```python
from build123d import *

# Parameters (mm, degrees)
SKETCH1_W           = 61
SKETCH1_H           = 10
SKETCH1_R           = 1.5
BOSS_EXTRUDE1_DEPTH = 5
SKETCH2_W           = 3
SKETCH2_H           = 10
BOSS_EXTRUDE2_DEPTH = 45
SKETCH3_R           = 1.75
CUT_EXTRUDE1_DEPTH  = 80.072172407
SKETCH4_W           = 15
SKETCH4_H           = 6
BOSS_EXTRUDE3_DEPTH = 3
SKETCH5_R           = 1.75
CUT_EXTRUDE2_DEPTH  = 82.52017035
SKETCH6_W           = 61
SKETCH6_H           = 10
SKETCH6_R           = 1.5
BOSS_EXTRUDE4_DEPTH = 5
SKETCH7_R           = 1.75
CUT_EXTRUDE3_DEPTH  = 85.679030308
SKETCH8_W           = 61
SKETCH8_H           = 55
SKETCH8_W_2         = 55
SKETCH8_H_2         = 45
BOSS_EXTRUDE5_DEPTH = 10
SKETCH13_R          = 1.7
CUT_EXTRUDE5_DEPTH  = 18


with BuildPart() as part:
    # Sketch1 → Boss-Extrude1 (new body)
    with BuildSketch(Plane(origin=(0, 0, 0), x_dir=(1, 0, 0), z_dir=(0, 1, 0))):
        with Locations((7.144615438, 0.604324155)):
            Rectangle(SKETCH1_W, SKETCH1_H)
        with Locations(Location((-17.855384562, 0.604324155, 0), (0, 0, 270))):
            Circle(SKETCH1_R, mode=Mode.SUBTRACT)
        with Locations(Location((-7.855384562, 0.604324155, 0), (0, 0, 270))):
            Circle(SKETCH1_R, mode=Mode.SUBTRACT)
        with Locations(Location((22.144615438, 0.604324155, 0), (0, 0, 270))):
            Circle(SKETCH1_R, mode=Mode.SUBTRACT)
        with Locations(Location((32.144615438, 0.604324155, 0), (0, 0, 270))):
            Circle(SKETCH1_R, mode=Mode.SUBTRACT)
    extrude(amount=BOSS_EXTRUDE1_DEPTH)

    # Sketch2 → Boss-Extrude2 (add)
    with BuildSketch(Plane(origin=(0, 5, 0), x_dir=(1, 0, 0), z_dir=(0, 1, 0))):
        with Locations((36.144615438, 0.604324155)):
            Rectangle(SKETCH2_W, SKETCH2_H)
        with Locations((-21.855384562, 0.604324155)):
            Rectangle(SKETCH2_W, SKETCH2_H)
    extrude(amount=BOSS_EXTRUDE2_DEPTH)

    # Sketch3 → Cut-Extrude1 (cut, through all)
    with BuildSketch(Plane.ZY.offset(23.355384562)):
        with Locations((-0.604324155, 10)):
            Circle(SKETCH3_R)
    extrude(amount=-CUT_EXTRUDE1_DEPTH, mode=Mode.SUBTRACT)

    # Sketch4 → Boss-Extrude3 (add)
    with BuildSketch(Plane.ZY.offset(23.355384562)):
        with Locations((-13.104324155, 24.14)):
            Rectangle(SKETCH4_W, SKETCH4_H)
    boss_extrude3 = extrude(amount=-BOSS_EXTRUDE3_DEPTH)

    # Mirror1: Boss-Extrude3 across plane
    add(boss_extrude3.mirror(Plane.ZY.offset(-7.144615438)))

    # Sketch5 → Cut-Extrude2 (cut, through all)
    with BuildSketch(Plane.ZY.offset(23.355384562)):
        with Locations((-14.744324155, 24.14)):
            Circle(SKETCH5_R)
    extrude(amount=-CUT_EXTRUDE2_DEPTH, mode=Mode.SUBTRACT)

    # Sketch6 → Boss-Extrude4 (add)
    with BuildSketch(Plane(origin=(0, 50, 0), x_dir=(1, 0, 0), z_dir=(0, 1, 0))):
        with Locations((7.144615438, 0.604324155)):
            Rectangle(SKETCH6_W, SKETCH6_H)
        with Locations(Location((2.144615438, 0.604324155, 0), (0, 0, 270))):
            Circle(SKETCH6_R, mode=Mode.SUBTRACT)
        with Locations(Location((12.144615438, 0.604324155, 0), (0, 0, 270))):
            Circle(SKETCH6_R, mode=Mode.SUBTRACT)
        with Locations(Location((-7.855384562, 0.604324155, 0), (0, 0, 270))):
            Circle(SKETCH6_R, mode=Mode.SUBTRACT)
        with Locations(Location((-17.855384562, 0.604324155, 0), (0, 0, 270))):
            Circle(SKETCH6_R, mode=Mode.SUBTRACT)
        with Locations(Location((22.144615438, 0.604324155, 0), (0, 0, 270))):
            Circle(SKETCH6_R, mode=Mode.SUBTRACT)
        with Locations(Location((32.144615438, 0.604324155, 0), (0, 0, 270))):
            Circle(SKETCH6_R, mode=Mode.SUBTRACT)
    extrude(amount=BOSS_EXTRUDE4_DEPTH)

    # Sketch7 → Cut-Extrude3 (cut, through all)
    with BuildSketch(Plane.ZY.offset(23.355384562)):
        with Locations((-0.604324155, 10)):
            Circle(SKETCH7_R)
        with Locations((-0.604324155, 20)):
            Circle(SKETCH7_R)
        with Locations((-0.604324155, 30)):
            Circle(SKETCH7_R)
        with Locations((-0.604324155, 40)):
            Circle(SKETCH7_R)
    extrude(amount=-CUT_EXTRUDE3_DEPTH, mode=Mode.SUBTRACT)

    # Sketch8 → Boss-Extrude5 (add)
    with BuildSketch(Plane.XY.offset(4.395675845)):
        with Locations((7.144615438, 27.5)):
            Rectangle(SKETCH8_W, SKETCH8_H)
        with Locations((7.144615438, 27.5)):
            Rectangle(SKETCH8_W_2, SKETCH8_H_2, mode=Mode.SUBTRACT)
    extrude(amount=BOSS_EXTRUDE5_DEPTH)

    # Sketch13 → Cut-Extrude5 (cut)
    with BuildSketch(Plane.XZ):
        with Locations(Location((-2.855384562, 9.395675845, 0), (0, 0, 270))):
            Circle(SKETCH13_R)
        with Locations(Location((-12.855384562, 9.395675845, 0), (0, 0, 270))):
            Circle(SKETCH13_R)
        with Locations(Location((17.144615438, 9.395675845, 0), (0, 0, 270))):
            Circle(SKETCH13_R)
        with Locations(Location((27.144615438, 9.395675845, 0), (0, 0, 270))):
            Circle(SKETCH13_R)
    extrude(amount=-CUT_EXTRUDE5_DEPTH, mode=Mode.SUBTRACT)


solid = part.part
```
Verification items for the finished model (mm, model axes). A direction names the side the tool comes from. Give positions to 0.01 mm unless a question says otherwise; leave off trailing zeros. Order: outer loops, then holes, each group sorted by start corner. A loop starts at its lowest first (then second) coordinate and runs counter-clockwise, first axis right, second up. Notation, with made-up numbers: (39.5, -1) -> (78.5, -1) arc R8 cw to (78.5, 11) -> close; hole circle Ø2 at (33, 5). An arc over 180 degrees is marked (long way). One line per item, written item: value.
(1) Tool access check on faces 5 (the face through (27.219, 2.465, 11.094)), 6 (the face through (20.68, 2.46, -0.93)). Record the directions out of +Z, -Z, +X, -X, +Y, -Y that give a thin tool (end or side, any length) a straight path to the whole face; none if there is none.
Final values:
face 5: -Y
face 6: +Y, -Y
(2) Sectioned sample at B-B on y = 24.14. Record the cut outline in (x, z), then the cut area to 3 significant figures.
Final values:
outline: (-23.36, -20.6) -> (-20.36, -20.6) -> (-20.36, -16.49) -> (-23.36, -16.49) -> close; (-23.36, -12.99) -> (-20.36, -12.99) -> (-20.36, 14.4) -> (-23.36, 14.4) -> close; (34.64, -20.6) -> (37.64, -20.6) -> (37.64, -16.49) -> (34.64, -16.49) -> close; (34.64, -12.99) -> (37.64, -12.99) -> (37.64, 14.4) -> (34.64, 14.4) -> close
area: 189 mm^2
(3) Sectioned sample at D-D on z = 12.5. Record the cut outline in (x, y).
Final values:
outline: (-23.36, 0) -> (37.64, 0) -> (37.64, 55) -> (-23.36, 55) -> close; hole (-20.36, 5) -> (34.64, 5) -> (34.64, 50) -> (-20.36, 50) -> close
(4) Sectioned sample at A-A on z = -17.5. Record the cut outline in (x, y), then the cut area to 3 significant figures.
Final values:
outline: (-23.36, 21.14) -> (-20.36, 21.14) -> (-20.36, 27.14) -> (-23.36, 27.14) -> close; (34.64, 21.14) -> (37.64, 21.14) -> (37.64, 27.14) -> (34.64, 27.14) -> close
area: 36.0 mm^2
(5) Scan lines: line 1 along X through (y, z) = (49.5, -1.5); line 2 along Y through (x, z) = (-19, 2.5). Record each from-to range of solid material in increasing order. Write a range as [from, to].
Final values:
line 1: [-23.36, -20.36], [34.64, 37.64]
line 2: [0, 5], [50, 55]
(6) Gauge pin test, flat end, axial feed: pin 1 (1.5 mm diameter, centred on x = 36.5, z = -10.5, fed in from -Y). Record the tip position at first contact, or that the pin passes through.
Final values:
pin 1: y = 21.14
(7) Sectioned sample at C-C on x = 7.5. Record the cut outline in (y, z), then the cut area to 3 significant figures.
Final values:
outline: (0, -5.6) -> (5, -5.6) -> (5, 14.4) -> (0, 14.4) -> close; (50, -5.6) -> (55, -5.6) -> (55, 14.4) -> (50, 14.4) -> close
area: 200 mm^2
(8) Draft check along Z on faces 1 (the face through (3.41, 52.46, 0.2)), 2 (the face through (34.645, 27, 4)), 3 (the face through (7, 51, -5.604)), 4 (the face through (-12.781, 2.465, 11.094)). Enter one of: pulls with the +Z half, pulls with the -Z half, needs draft (parallel to the pull), parting line crosses it, or undercut.
Final values:
face 1: undercut
face 2: needs draft
face 3: pulls with the -Z half
face 4: undercut
